```python
from build123d import *

# Parameters (mm, degrees)
SKETCH1_R           = 12.25
BOSS_EXTRUDE1_DEPTH = 18
SKETCH2_R           = 6.35
CUT_EXTRUDE1_DEPTH  = 40


with BuildPart() as part:
    # Sketch1 → Boss-Extrude1 (new body)
    with BuildSketch(Plane(origin=(0, 0, 0), x_dir=(0, 0, -1), z_dir=(1, 0, 0))):
        Polygon((0, 0), (0, 605), (180, 605), (180, 592), (1305, 400), (1305, 0), align=None)
        with Locations((1216, 365.189333333)):
            Circle(SKETCH1_R, mode=Mode.SUBTRACT)
        with Locations((1170, 373.04)):
            Circle(SKETCH1_R, mode=Mode.SUBTRACT)
    extrude(amount=BOSS_EXTRUDE1_DEPTH)

    # Sketch2 → Cut-Extrude1 (cut)
    with BuildSketch(Plane(origin=(18, 0, 0), x_dir=(0, 0, -1), z_dir=(1, 0, 0))):
        with Locations((241.3, 516.1)):
            Circle(SKETCH2_R)
    extrude(amount=-CUT_EXTRUDE1_DEPTH, mode=Mode.SUBTRACT)


solid = part.part
```
Geometry check sheet. Reference: the model listing, model coordinates, mm. Coordinates: 2 decimals unless noted, no trailing zeros. Order: outer loops, then holes, each group sorted by start corner. A loop starts at its lowest first (then second) coordinate and runs counter-clockwise, first axis right, second up.
Item 1: Section check C-C (z = -335). Enter the section's corners in (x, y).
Item 2: Section check B-B (x = 10). Enter the section's corners in (y, z).
Item 3: Mould release check, pull along Y, two halves, no side actions. Record for faces 1 (the flat face through (0, 240, -662)), 2 (the flat face through (8.874, 497.344, -734.625)), 3 (the cylindrical face through (8.87, 353.23, -1213.34)): released by +Y, released by -Y, zero draft, split by the parting line, or undercut.
Item 4: Section check D-D (z = -198.5). Enter the section's corners in (x, y), plus the area to 3 significant figures.
Item 5: Depth check by flat-ended pin: pin 1 (6.5 mm diameter, centred on x = 7, y = 595.5, fed in from -Z). Enter the tip coordinate at first touch or a pass-through.
Item 6: Section check A-A (z = -1216). Enter the section's corners in (x, y).
Item 7: Scan lines: line 1 along Y through (x, z) = (8.5, -1216); line 2 along Y through (x, z) = (7.5, -1170); line 3 along Y through (x, z) = (12.75, -592.5). Record each from-to range of solid material in increasing order.
Check sheet entries:
1. outline: (0, 0) - (18, 0) - (18, 565.55) - (0, 565.55) - close
2. outline: (0, -1305) - (400, -1305) - (592, -180) - (605, -180) - (605, 0) - (0, 0) - close; hole circle Ø24.5 at (365.19, -1216); hole circle Ø24.5 at (373.04, -1170); hole circle Ø12.7 at (516.1, -241.3)
3. face 1: zero draft
3. face 2: released by +Y
3. face 3: undercut
4. outline: (0, 0) - (18, 0) - (18, 588.84) - (0, 588.84) - close
4. area: 10,600 mm2
5. pin 1: stops at z = -180
6. outline: (0, 0) - (18, 0) - (18, 352.94) - (0, 352.94) - close; (0, 377.44) - (18, 377.44) - (18, 415.19) - (0, 415.19) - close
7. line 1: y = 0 to 352.94, 377.44 to 415.19
7. line 2: y = 0 to 360.79, 385.29 to 423.04
7. line 3: y = 0 to 521.6
